Here's how the part is built. I have some questions about the finished solid (model axes, mm). A direction names the side the tool comes from. Give positions to 0.01 mm unless a question says otherwise; leave off trailing zeros. Write each loop counter-clockwise with the first axis right and the second up, starting at its lowest first coordinate (ties: lowest second). Pieces come first, ordered by that corner, then holes. Notation, with made-up numbers: (52.5, 68) -> (82.5, 68) arc R33 ccw to (82.5, 97) -> close; hole circle Ø9 at (43.25, 29.5). An arc over 180 degrees is marked (long way). Use CSV: the item, a comma, the result in double quotes. Start each with the question number.
(1) If we mould it in two halves opening along X, with no side actions, what happens to faces 1 (the cylindrical face through (-3.102, 1.192, 1.621)), 2 (the flat face through (0.1, 8.5, -2.4)), 3 (the cylindrical face through (-9.76, 4.08, -2.17))? For each: pulls with the +X half, pulls with the -X half, needs draft (parallel to the pull), parting line crosses it, or undercut.
(2) Suppose I cut it at D-D on z = 6.25. List the corners of the cut face in (x, y) for me, plus the area to 3 significant figures.
(3) For pin 1 Ø1.5 at (x, z) = (-7, -7.5) entering from -Y; pin 2 Ø3 at (x, y) = (3, 1.5) entering from -Z; pin 3 Ø5.5 at (x, z) = (-1, -1) entering from -Y; pin 4 Ø4 at (x, z) = (0, 0) entering from +Y, each with a flat end and sliding along its axis, tell me the tip position at first contact or that it passes through.
(4) Suppose I cut it at B-B on x = -0.5. List the corners of the cut face in (y, z) for me, plus the area to 3 significant figures.
(5) Which directions (+Z, -Z, +X, -X, +Y, -Y) give clear straight access to the entire face, cutting with the end or side of a thin tool? Please do faces 4 (the cylindrical face through (-0.37, 4.22, -6.11)), 5 (the flat face through (0.3, 2.378, 2.3)).
(6) Suppose I cut it at A-A on z = 0. List the corners of the cut face in (x, y) for me.
(7) Suppose I cut it at C-C on y = 4.25. List the corners of the cut face in (x, z) for me, plus the area to 3 significant figures.
(8) I need wall thicknesses on L1, parallel to X at y = 4.5, z = 0; L2, parallel to X at y = 1.7, z = 0; L3, parallel to Y at x = -2.25, z = -0.25. Which ranges of each line are inside material? Lowest first, please. Write a range as [from, to].
from build123d import *

# Parameters (mm, degrees)
BOSS_EXTRUDE1_DEPTH      = 8.5
BOSS_EXTRUDE1_DEPTH_BACK = 2
SKETCH1_R                = 10
SKETCH3_W                = 3.5
SKETCH3_H                = 2.6
SKETCH4_R                = 2.1
CUT_EXTRUDE1_DEPTH       = 17.615368622
SKETCH5_R                = 1.5
CUT_EXTRUDE2_DEPTH       = 17.615368622


with BuildPart() as part:
    # Sketch1 → Boss-Extrude1 (new, two sides: drawn at the far end of the back side and taken through both)
    with BuildSketch(Plane(origin=(0, 0, 0), x_dir=(1, 0, 0), z_dir=(0, 1, 0)).offset(-BOSS_EXTRUDE1_DEPTH_BACK)):
        with Locations(Location((0, 0, 0), (0, 0, 270))):
            Circle(SKETCH1_R)
    extrude(amount=BOSS_EXTRUDE1_DEPTH + BOSS_EXTRUDE1_DEPTH_BACK)

    # Sketch2 → Cut-Revolve1 (revolve, cut)
    with BuildSketch(Plane(origin=(0, 0, 0), x_dir=(0, 0, -1), z_dir=(1, 0, 0))):
        with BuildLine():
            Line((0, 0), (0, -451))
            ThreePointArc((0, -451), (-225.5, -225.5), (0, 0))
        make_face()
    revolve(axis=Axis((0, 0, 0), (0, -1, 0)), mode=Mode.SUBTRACT)

    # Sketch3 → Cut-Revolve2 (revolve, cut)
    with BuildSketch(Plane(origin=(0, 0, 0), x_dir=(0, 0, -1), z_dir=(1, 0, 0)), mode=Mode.PRIVATE) as cut_revolve2_sk:
        with Locations((-1.75, 1.078161392)):
            Rectangle(SKETCH3_W, SKETCH3_H)
    revolve(cut_revolve2_sk.sketch.rotate(Axis((0, 2.378161392, 0), (0, -1, 0)), 84.935699762), axis=Axis((0, 2.378161392, 0), (0, -1, 0)), mode=Mode.SUBTRACT)

    # Sketch4 → Cut-Extrude1 (cut, through all)
    with BuildSketch(Plane(origin=(0, 8.5, 0), x_dir=(1, 0, 0), z_dir=(0, 1, 0))):
        with Locations(Location((0, 0, 0), (0, 0, 270))):
            Circle(SKETCH4_R)
    extrude(amount=-CUT_EXTRUDE1_DEPTH, mode=Mode.SUBTRACT)

    # Sketch5 → Cut-Extrude2 (cut, through all)
    with BuildSketch(Plane(origin=(0, 8.5, 0), x_dir=(1, 0, 0), z_dir=(0, 1, 0))):
        with Locations(Location((0.20360383, 7.497235856, 0), (0, 0, 270))):
            Circle(SKETCH5_R)
        with Locations(Location((4.24204571, -6.185066547, 0), (0, 0, 270))):
            Circle(SKETCH5_R)
    extrude(amount=-CUT_EXTRUDE2_DEPTH, mode=Mode.SUBTRACT)


solid = part.part
Geometry says:
1,face 1,"undercut"
1,face 2,"needs draft"
1,face 3,"parting line crosses it"
2,outline,"(-7.81, -0.22) arc R225.41 cw to (2.74, -0.1) -> (2.74, 8.5) -> (-7.81, 8.5) -> close; (5.74, -0.16) arc R225.41 cw to (7.81, -0.22) -> (7.81, 8.5) -> (5.74, 8.5) -> close"
2,area,"109 mm²"
3,pin 1,"y = -0.22"
3,pin 2,"z = -9.89"
3,pin 3,"y = -0.04"
3,pin 4,"through"
4,outline,"(-0.22, -9.99) -> (8.5, -9.99) -> (8.5, -8.82) -> (-0.17, -8.82) arc R225.5 cw to start; (-0.22, 9.99) arc R225.5 cw to (-0.03, 3.46) -> (2.38, 3.46) -> (2.38, 2.04) -> (8.5, 2.04) -> (8.5, 9.99) -> close; (-0.09, -6.17) -> (8.5, -6.17) -> (8.5, -2.04) -> (2.38, -2.04) -> (2.38, -3.46) -> (-0.03, -3.46) arc R225.5 cw to start"
4,area,"107 mm²"
5,face 4,"+Y, -Y"
5,face 5,"-Y"
6,outline,"(-10, -0.22) arc R225.5 cw to (-3.5, -0.03) -> (-3.5, 2.38) -> (-2.1, 2.38) -> (-2.1, 8.5) -> (-10, 8.5) -> close; (2.1, 2.38) -> (3.5, 2.38) -> (3.5, -0.03) arc R225.5 cw to (10, -0.22) -> (10, 8.5) -> (2.1, 8.5) -> close"
7,outline,"circle Ø20 at (0, 0); hole circle Ø4.2 at (0, 0); hole circle Ø3 at (0.2, -7.5); hole circle Ø3 at (4.24, 6.19)"
7,area,"286 mm²"
8,L1,"[-10, -2.1], [2.1, 10]"
8,L2,"[-10, -3.5], [3.5, 10]"
8,L3,"[2.38, 8.5]"
